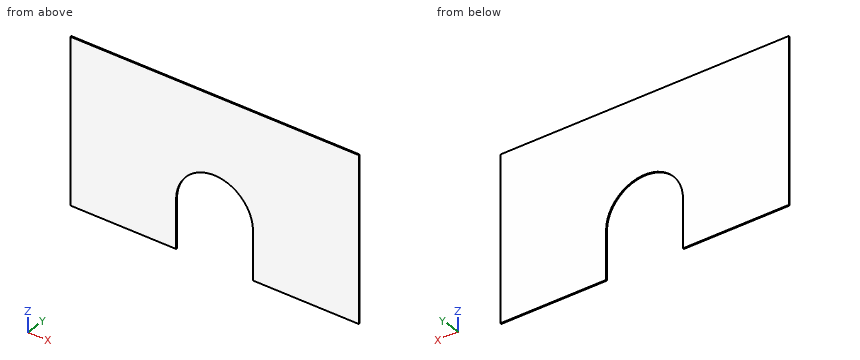
from build123d import *

# Parameters (mm, degrees)
F1_DEPTH = 3.175


# Not quite as in the source:
# - a length typed as a fraction of an inch, garbled in the dataset ("3 / 203.2 mm" for 3/8 in), is restored


with BuildPart() as f1:
    # F0 (on Front) → F1 (new body)
    with BuildSketch(Plane.XZ):
        with BuildLine():
            Line((381, -215.9), (381, 215.9))
            Line((381, 215.9), (-381, 215.9))
            Line((-381, 215.9), (-381, -215.9))
            Line((-381, -215.9), (-101.6, -215.9))
            Line((-101.6, -215.9), (-101.6, -88.9))
            ThreePointArc((-101.6, -88.9), (0, 12.7), (101.6, -88.9))
            Line((101.6, -88.9), (101.6, -215.9))
            Line((101.6, -215.9), (381, -215.9))
        make_face()
    extrude(amount=F1_DEPTH)


solid = f1.part
The listing builds one solid part. Answer for the finished solid, in the listing's coordinates (mm). Give positions to 0.01 mm unless a question says otherwise; leave off trailing zeros. Write each loop counter-clockwise with the first axis right and the second up, starting at its lowest first coordinate (ties: lowest second). Pieces come first, ordered by that corner, then holes.
1) Find the intervals of material crossed by L1, parallel to X at y = -0.45, z = -160; L2, parallel to Z at x = -4.5, y = -0.9; L3, parallel to X at y = -2.55, z = -41.5, in increasing order.
2) Section A-A (y = -1.2) is taken. Write down the section's boundary in (x, z).
3) Section B-B (x = 0) is taken. Write down the section's boundary in (y, z) (3 decimals), and give its area (3 significant figures).
Response:
1. L1: x = -381 to -101.6, 101.6 to 381
1. L2: z = 12.6 to 215.9
1. L3: x = -381 to -89.87, 89.87 to 381
2. outline: (-381, -215.9) - (-101.6, -215.9) - (-101.6, -88.9) arc R101.6 cw to (101.6, -88.9) - (101.6, -215.9) - (381, -215.9) - (381, 215.9) - (-381, 215.9) - close
3. outline: (-3.175, 12.7) - (0, 12.7) - (0, 215.9) - (-3.175, 215.9) - close
3. area: 645 mm2
